Can you work these out from the model? Positions are in its coordinate system, mm. A direction names the side the tool comes from. Coordinates: 2 decimals unless noted, no trailing zeros. Order: outer loops, then holes, each group sorted by start corner. A loop starts at its lowest first (then second) coordinate and runs counter-clockwise, first axis right, second up. Notation, with made-up numbers: (-36.5, 54.25) -> (6.5, 54.25) arc R15 cw to (6.5, 60.25) -> close; hole circle Ø5 at (-12, 54). An arc over 180 degrees is marked (long way). Use a Markdown table: item, result. Add a question column.
1. Suppose I cut it at D-D, the plane y = -10. List the corners of the cut face in (x, z) for me, then the cut area to 3 significant figures.
2. Suppose I cut it at A-A, the plane y = 15.5. List the corners of the cut face in (x, z) for me.
3. For faces 5 (the flat face through (-20, -20, -17)), 6 (the flat face through (-10, 10, 0)), which set-ups out of +Z, -Z, +X, -X, +Y, -Y let a thin tool reach every point of the face, with its end or its side?
4. Suppose I cut it at B-B, the plane z = -20. List the corners of the cut face in (x, y) for me.
5. For pin 1 Ø6 at (x, y) = (-11.5, -7.5) entering from +Z; pin 2 Ø12 at (y, z) = (-1.5, 13) entering from +X; pin 3 Ø3 at (x, y) = (16, 6.5) entering from +Z; pin 4 Ø1.8 at (x, y) = (-15.5, -15.5) entering from +Z, each with a flat end and sliding along its axis, tell me the tip position at first contact or that it passes through.
6. If I drill on line 1 along Y through (x, z) = (-15.5, -25.5); line 2 along Y through (x, z) = (15, -11); line 3 along Z through (x, y) = (0.5, -12), over which ranges is the centre line in solid material (lowest first)? Write a range as from..to.
7. We'd pull the mould along Y, two halves only. Please class faces 1 (the flat face through (0, -21, -17)), 2 (the cylindrical face through (14, -15.43, -16.76)), 3 (the cylindrical face through (14, 15.57, -16.76)), 4 (the flat face through (20, 20, -17)): pulls with the +Y half, pulls with the -Y half, needs draft (parallel to the pull), parting line crosses it, or undercut.
```python
from build123d import *

# Parameters (mm, degrees)
SKETCH_1_W      = 42
SKETCH_1_H      = 42
SKETCH_1_R      = 1.5
SKETCH_1_R_2    = 11
SKETCH_1_R_3    = 2.5
EXTRUDE_1_DEPTH = 34
SKETCH_1_3_R    = 11
SKETCH_1_3_R_2  = 2.5
EXTRUDE_2_DEPTH = 2
SKETCH_1_4_R    = 2.5
EXTRUDE_3_DEPTH = 22
CHAMFER_1_SIZE  = 2


with BuildPart() as part:
    # Sketch 1 → Extrude 1 (new body)
    # profile 1 of 3: a face of its own
    with BuildSketch(Plane.XY):
        Rectangle(SKETCH_1_W, SKETCH_1_H)
        with Locations((15.5, -15.5)):
            Circle(SKETCH_1_R, mode=Mode.SUBTRACT)
        with Locations((-15.5, -15.5)):
            Circle(SKETCH_1_R, mode=Mode.SUBTRACT)
        with Locations((-15.5, 15.5)):
            Circle(SKETCH_1_R, mode=Mode.SUBTRACT)
        with Locations((15.5, 15.5)):
            Circle(SKETCH_1_R, mode=Mode.SUBTRACT)
        Circle(SKETCH_1_R_2, mode=Mode.SUBTRACT)
    # profile 2 of 3: a face of its own
    with BuildSketch(Plane.XY):
        Circle(SKETCH_1_R_2)
        Circle(SKETCH_1_R_3, mode=Mode.SUBTRACT)
    # profile 3 of 3: a face of its own
    with BuildSketch(Plane.XY):
        Circle(SKETCH_1_R_3)
    extrude(amount=-EXTRUDE_1_DEPTH)

    # Sketch 1_3 → Extrude 2 (add)
    # profile 1 of 2: a face of its own
    with BuildSketch(Plane.XY):
        Circle(SKETCH_1_3_R)
        Circle(SKETCH_1_3_R_2, mode=Mode.SUBTRACT)
    # profile 2 of 2: a face of its own
    with BuildSketch(Plane.XY):
        Circle(SKETCH_1_3_R_2)
    extrude(amount=EXTRUDE_2_DEPTH)

    # Sketch 1_4 → Extrude 3 (add)
    with BuildSketch(Plane.XY):
        Circle(SKETCH_1_4_R)
    extrude(amount=EXTRUDE_3_DEPTH)

    # Chamfer 1
    chamfer_1_edges = [part.edges().sort_by_distance(p)[0] for p in [
        (21, -21, -17),
        (-21, -21, -17),
        (-21, 21, -17),
        (21, 21, -17),
    ]]
    chamfer(chamfer_1_edges, length=CHAMFER_1_SIZE)


solid = part.part
```
Worked out:
| question | item | result |
|---|---|---|
| 1 | outline | (-21, -34) -> (21, -34) -> (21, 0) -> (4.58, 0) -> (4.58, 2) -> (-4.58, 2) -> (-4.58, 0) -> (-21, 0) -> close |
| 1 | area | 1,450 mm² |
| 2 | outline | (-21, -34) -> (-17, -34) -> (-17, 0) -> (-21, 0) -> close; (-14, -34) -> (14, -34) -> (14, 0) -> (-14, 0) -> close; (17, -34) -> (21, -34) -> (21, 0) -> (17, 0) -> close |
| 3 | face 5 | +Z, -Z, -X, -Y |
| 3 | face 6 | +Z |
| 4 | outline | (-21, -19) -> (-19, -21) -> (19, -21) -> (21, -19) -> (21, 19) -> (19, 21) -> (-19, 21) -> (-21, 19) -> close; hole circle Ø3 at (-15.5, -15.5); hole circle Ø3 at (-15.5, 15.5); hole circle Ø3 at (15.5, -15.5); hole circle Ø3 at (15.5, 15.5) |
| 5 | pin 1 | stops at z = 2 |
| 5 | pin 2 | stops at x = 2.5 |
| 5 | pin 3 | stops at z = 0 |
| 5 | pin 4 | passes through |
| 6 | line 1 | y = -21..-17, -14..14, 17..21 |
| 6 | line 2 | y = -21..-16.91, -14.09..14.09, 16.91..21 |
| 6 | line 3 | z = -34..0 |
| 7 | face 1 | pulls with the -Y half |
| 7 | face 2 | undercut |
| 7 | face 3 | undercut |
| 7 | face 4 | pulls with the +Y half |
